Print and shaded views of the part. All mm, measured from the part's lowest x, y and z. Round coordinates to 2 decimals unless told otherwise and drop trailing zeros. Write each loop counter-clockwise with the first axis right and the second up, starting at its lowest first coordinate (ties: lowest second). Pieces come first, ordered by that corner, then holes. Notation, with made-up numbers: (87.25, -8) - (141.25, -8) arc R5 ccw to (141.25, 1) - close; hole circle Ø8 at (8, 72.25). An arc over 180 degrees is marked (long way). One line per item, written item: value.
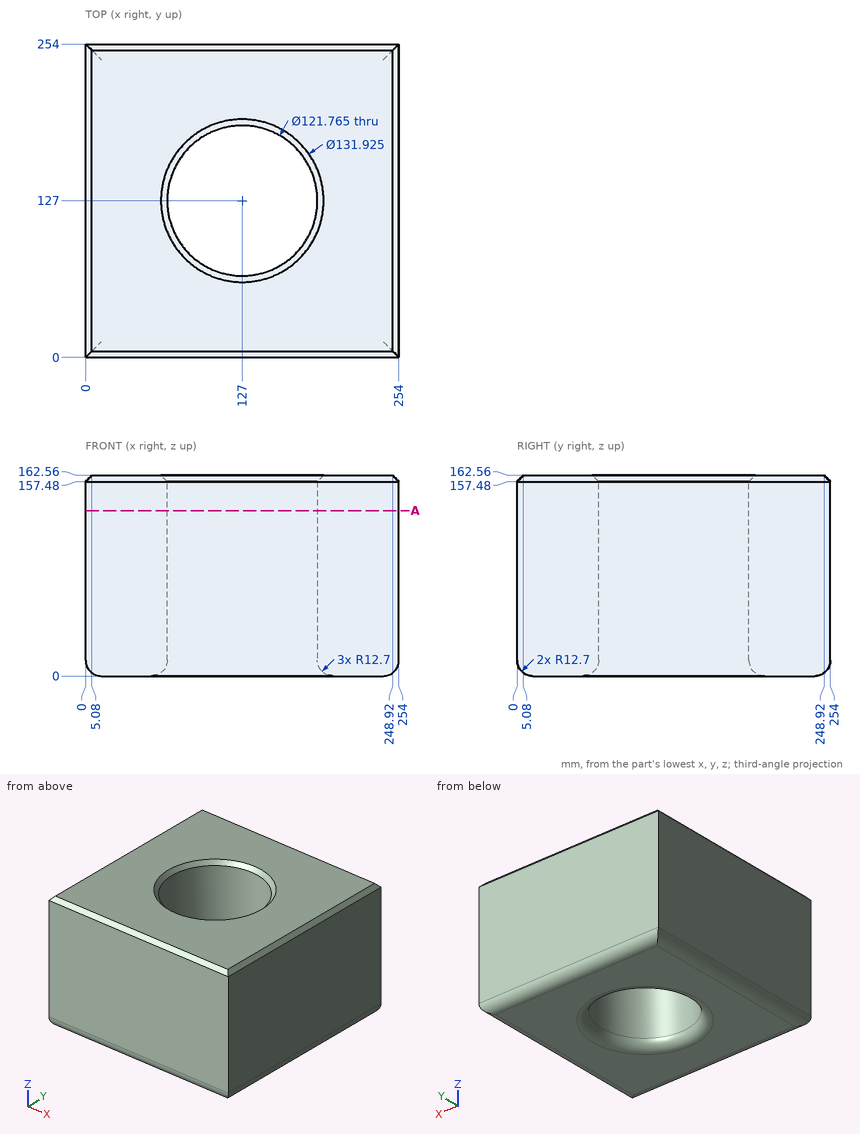
1. Wall check: probe 1 along Y at (x, z) = (127, 126.5); probe 2 along X at (y, z) = (172, 29.5); probe 3 along X at (y, z) = (140.5, 104.5). Give the ranges that are in metal, low to high. Write a range as [from, to].
Report:
probe 1: [0, 66.12], [187.88, 254]
probe 2: [0, 85.99], [168.01, 254]
probe 3: [0, 67.63], [186.37, 254]
2. Band-saw the part on A-A on z = 134. Write the cut outline in (x, y) (1 decimal).
Report:
outline: (0, 0) - (254, 0) - (254, 254) - (0, 254) - close; hole circle Ø121.8 at (127, 127)
3. Drop a flat-ended pin along its axis: pin 1 (5 mm diameter, centred on x = 102, y = 188.5, fed in from -Z). Give the stop position or say it passes through.
Report:
pin 1: z = 0.9
